from build123d import *

# Parameters (mm, degrees)
ESKIZ_KONTUR_W        = 12.6
ESKIZ_KONTUR_H        = 23.2
PLASTINA_DEPTH        = 3
OTVERSTIYA_DEPTH      = 37.523967755
OTVERSTIYA_DEPTH_BACK = 37.523967755
ESKIZ_OTVERSTIYA_R    = 1.65
ESKIZ_OTVERSTIYA_R_2  = 1.1


with BuildPart() as part:
    # Eskiz_kontur → Plastina (new body)
    with BuildSketch(Plane.XY):
        with BuildLine():
            Line((-19.608453592, 2.472140862), (-12.657403592, 24.163120862))
            ThreePointArc((-12.657403592, 24.163120862), (-10.114503963, 27.663122227), (-6.000005728, 29.000003803))
            Line((-6.000005728, 29.000003803), (5.999994272, 29.000003803))
            ThreePointArc((5.999994272, 29.000003803), (9.420342449, 28.10747607), (11.968474679, 25.657494531))
            Line((11.968474679, 25.657494531), (19.542154679, 13.396244531))
            ThreePointArc((19.542154679, 13.396244531), (20.190566029, 11.981622791), (20.484159934, 10.453423012))
            Line((20.484159934, 10.453423012), (21.999989934, -11.999996988))
            Line((21.999989934, -11.999996988), (21.999989934, -22))
            Line((21.999989934, -22), (16, -22))
            Line((16, -22), (16, -25))
            Line((16, -25), (6, -25))
            Line((6, -25), (6, -22))
            Line((6, -22), (1.65, -22))
            Line((1.65, -22), (1.65, -17.5))
            Line((1.65, -17.5), (2.9, -17.5))
            Line((2.9, -17.5), (2.9, -14.9))
            Line((2.9, -14.9), (1.65, -14.9))
            Line((1.65, -14.9), (1.65, -12))
            Line((1.65, -12), (-1.65, -12))
            Line((-1.65, -12), (-1.65, -14.9))
            Line((-1.65, -14.9), (-2.9, -14.9))
            Line((-2.9, -14.9), (-2.9, -17.5))
            Line((-2.9, -17.5), (-1.65, -17.5))
            Line((-1.65, -17.5), (-1.65, -22))
            Line((-1.65, -22), (-6, -22))
            Line((-6, -22), (-6, -25))
            Line((-6, -25), (-16, -25))
            Line((-16, -25), (-16, -22))
            Line((-16, -22), (-22, -22))
            Line((-22, -22), (-22, -12))
            Line((-22, -12), (-19.90151, 1.25148))
            ThreePointArc((-19.90151, 1.25148), (-19.778961323, 1.867567439), (-19.608453592, 2.472140862))
        make_face()
        with Locations((12, -5.4)):
            Rectangle(ESKIZ_KONTUR_W, ESKIZ_KONTUR_H, mode=Mode.SUBTRACT)
    extrude(amount=PLASTINA_DEPTH)

    # Eskiz_otverstiya → Otverstiya (cut, two sides: drawn at the far end of the back side and taken through both)
    with BuildSketch(Plane.XY.offset(-OTVERSTIYA_DEPTH_BACK)):
        with Locations((-12, 0)):
            Circle(ESKIZ_OTVERSTIYA_R)
        with Locations((12, -19.3)):
            Circle(ESKIZ_OTVERSTIYA_R_2)
        with Locations((-6, 22)):
            Circle(ESKIZ_OTVERSTIYA_R)
        with Locations((12, 8.5)):
            Circle(ESKIZ_OTVERSTIYA_R_2)
        with Locations((6, 22)):
            Circle(ESKIZ_OTVERSTIYA_R)
    extrude(amount=OTVERSTIYA_DEPTH + OTVERSTIYA_DEPTH_BACK, mode=Mode.SUBTRACT)


solid = part.part
The listing builds one solid part. Answer for the finished solid, in the listing's coordinates (mm). A direction names the side the tool comes from. Round coordinates to 2 decimals unless told otherwise and drop trailing zeros. Order: outer loops, then holes, each group sorted by start corner. A loop starts at its lowest first (then second) coordinate and runs counter-clockwise, first axis right, second up. Notation, with made-up numbers: (45.25, 57) - (53.25, 57) arc R17 cw to (53.25, 85) - close; hole circle Ø4 at (62.25, 78). An arc over 180 degrees is marked (long way). Write item = value, one per line. Start each with the question number.
1) For faces 4 (the flat face through (-19, -22, 1)), 5 (the flat face through (-2, -14.9, 1)), 6 (the flat face through (-1.65, -20, 1)), determine the directions among +Z, -Z, +X, -X, +Y, -Y from which every point of the face is accessible in a straight line to the end or side of a thin tool.
2) Straight lines are drawn through the part: L1, parallel to X at y = -1, z = 2.1; L2, parallel to Y at x = 12, z = 1.95; L3, parallel to X at y = 22, z = 1.75. For each, find the intervals that lie inside material, in ascending order.
3) Section A-A, the plane y = -19.3 is taken. Write down the section's boundary in (x, z), plus the area to 4 significant figures.
4) Given pin 1 (1.5 mm diameter, centred on y = -24, z = 1.5, fed in from -X); pin 2 (3 mm diameter, centred on x = -6, y = 22, fed in from -Z); pin 3 (1.5 mm diameter, centred on y = 4, z = 1, fed in from +X); pin 4 (0.9 mm diameter, centred on y = -8.5, z = 1, fed in from +X), each flat-ended and moving along its own axis, determine where each tip first touches the part or whether it passes through.
5) Section C-C, the plane x = 10 is taken. Write down the section's boundary in (y, z).
6) Section B-B, the plane y = -11 is taken. Write down the section's boundary in (x, z), plus the area to 3 significant figures.
7) Section D-D, the plane z = 0.9 is taken. Count the separate pieces of the cut face and the enclosed holes in it, plus the area to 3 significant figures.
8) For a pull along X with two mould halves and no side action, classify faces 1 (the flat face through (-11, -25, 1)), 2 (the cylindrical face through (13.016, 8.079, 1.479)), 3 (the flat face through (16, -23, 1)) as released by +X, released by -X, zero draft, split by the parting line, or undercut.
Results list:
q1.face_4 = +Z, -Z, -X, -Y
q1.face_5 = +Z, -Z
q1.face_6 = +Z, -Z, -Y
q2.L1 = -20.26 to -13.31, -10.69 to 5.7, 18.3 to 21.26
q2.L2 = -25 to -20.4, -18.2 to -17, 6.2 to 7.4, 9.6 to 25.61
q2.L3 = -13.35 to -7.65, -4.35 to 4.35, 7.65 to 14.23
q3.outline = (-22, 0) - (-1.65, 0) - (-1.65, 3) - (-22, 3) - close; (1.65, 0) - (10.9, 0) - (10.9, 3) - (1.65, 3) - close; (13.1, 0) - (22, 0) - (22, 3) - (13.1, 3) - close
q3.area = 115.5 mm^2
q4.pin_1 = -16
q4.pin_2 = through
q4.pin_3 = 20.97
q4.pin_4 = 21.79
q5.outline = (-25, 0) - (-17, 0) - (-17, 3) - (-25, 3) - close; (6.2, 0) - (27.74, 0) - (27.74, 3) - (6.2, 3) - close
q6.outline = (-21.84, 0) - (5.7, 0) - (5.7, 3) - (-21.84, 3) - close; (18.3, 0) - (21.93, 0) - (21.93, 3) - (18.3, 3) - close
q6.area = 93.5 mm^2
q7.separate_pieces = 1
q7.enclosed_holes = 6
q7.area = 1,600 mm^2
q8.face_1 = zero draft
q8.face_2 = undercut
q8.face_3 = released by +X
